```python
from build123d import *

# Parameters (mm, degrees)
ESQUISSE1_W             = 70
ESQUISSE1_H             = 30
BOSS_EXTRU_1_DEPTH      = 10
ESQUISSE2_R             = 0.8
ENL_V_MAT_EXTRU_1_DEPTH = 77.811457479
ESQUISSE3_R             = 1.025
ENL_V_MAT_EXTRU_2_DEPTH = 77.811457622
CONG_2_R                = 20


with BuildPart() as part:
    # Esquisse1 → Boss.-Extru.1 (new body)
    with BuildSketch(Plane.XY):
        with Locations((35, 15)):
            Rectangle(ESQUISSE1_W, ESQUISSE1_H)
    extrude(amount=BOSS_EXTRU_1_DEPTH)

    # Esquisse2 → Enlèv. mat.-Extru.1 (cut, through all)
    with BuildSketch(Plane.XY.offset(10)):
        with Locations((53.974554028, 20.976947928)):
            Circle(ESQUISSE2_R)
        with Locations((59.413465757, 18.443523524)):
            Circle(ESQUISSE2_R)
        with Locations((59.938911728, 12.466575596)):
            Circle(ESQUISSE2_R)
        with Locations((55.025445972, 9.023052072)):
            Circle(ESQUISSE2_R)
        with BuildLine():
            ThreePointArc((54.940833126, 19.980528702), (59.5, 15), (54.940833126, 10.019471298))
            add(Edge.make_bspline(
                [(48.86, 7.668533571), (51.540343022, 10.446024006), (54.940833126, 10.019471298)],
                knots=[0, 0, 0, 1, 1, 1], degree=2))
            ThreePointArc((48.86, 7.668533571), (28.5, 15), (48.86, 22.331466429))
            add(Edge.make_bspline(
                [(48.86, 22.331466429), (51.534478996, 19.459310032), (54.940833126, 19.980528702)],
                knots=[0, 0, 0, 1, 1, 1], degree=2))
        make_face()
    extrude(amount=-ENL_V_MAT_EXTRU_1_DEPTH, mode=Mode.SUBTRACT)

    # Esquisse3 → Enlèv. mat.-Extru.2 (cut, through all)
    with BuildSketch(Plane.XY.offset(10)):
        with Locations((5, 25)):
            Circle(ESQUISSE3_R)
        with Locations((65.771138483, 5)):
            Circle(ESQUISSE3_R)
        with Locations((65, 25)):
            Circle(ESQUISSE3_R)
    extrude(amount=-ENL_V_MAT_EXTRU_2_DEPTH, mode=Mode.SUBTRACT)

    # Congé2
    cong_2_edges = [part.edges().sort_by_distance(p)[0] for p in [
        (0, 0, 5),
    ]]
    fillet(cong_2_edges, radius=CONG_2_R)


solid = part.part
```
Part model, mm, in its own coordinate system. A direction names the side the tool comes from. Round coordinates to 2 decimals unless told otherwise and drop trailing zeros. Write each loop counter-clockwise with the first axis right and the second up, starting at its lowest first coordinate (ties: lowest second). Pieces come first, ordered by that corner, then holes.
Item 1: Which spindle directions (+Z, -Z, +X, -X, +Y, -Y) get a long thin tool onto all of the face, cutting with end or side? Do faces 1 (the cylindrical face through (59.5, 15.1, 5.1)), 2 (the flat face through (45, 0, 5)). Say none if no direction does.
Results:
face 1: +Z, -Z
face 2: +Z, -Z, +X, -X, -Y
Item 2: Cut at D-D, the plane y = 15. Give the cut face in (x, z), plus the area to 3 significant figures.
Results:
outline: (0.64, 0) - (28.5, 0) - (28.5, 10) - (0.64, 10) - close; (59.5, 0) - (70, 0) - (70, 10) - (59.5, 10) - close
area: 384 mm2
Item 3: Drop flat-ended pins along their axis: pin 1 Ø3 at (y, z) = (14, 6) entering from -X; pin 2 Ø1.3 at (x, y) = (55.03, 9.02) entering from -Z. Give the stop position or say it passes through.
Results:
pin 1: stops at x = 0.51
pin 2: passes through
Item 4: Probe L1, parallel to X at y = 21.5, z = 2.25; L2, parallel to X at y = 19.5, z = 9.25; L3, parallel to Y at x = 30, z = 8. List the from-to ranges inside material, lowest first.
Results:
L1: x = 0 to 30.51, 49.73 to 53.37, 54.58 to 70
L2: x = 0.01 to 29.42, 56.68 to 70
L3: y = 0 to 9.32, 20.68 to 30
Item 5: Cut at A-A, the plane x = 40. Give the cut face in (y, z).
Results:
outline: (0, 0) - (3.5, 0) - (3.5, 10) - (0, 10) - close; (26.5, 0) - (30, 0) - (30, 10) - (26.5, 10) - close
Item 6: Cut at C-C, the plane y = 25. Give the cut face in (x, z) (3 decimals), plus the area to 3 significant figures.
Results:
outline: (0, 0) - (3.975, 0) - (3.975, 10) - (0, 10) - close; (6.025, 0) - (34.321, 0) - (34.321, 10) - (6.025, 10) - close; (45.679, 0) - (63.975, 0) - (63.975, 10) - (45.679, 10) - close; (66.025, 0) - (70, 0) - (70, 10) - (66.025, 10) - close
area: 545 mm2
Item 7: Cut at B-B, the plane y = 5. Give the cut face in (x, z).
Results:
outline: (6.77, 0) - (34.32, 0) - (34.32, 10) - (6.77, 10) - close; (45.68, 0) - (64.75, 0) - (64.75, 10) - (45.68, 10) - close; (66.8, 0) - (70, 0) - (70, 10) - (66.8, 10) - close
Item 8: Two-plate mould, pull along X, no slides. Class faces 3 (the cylindrical face through (5.703, 6.014, 5.07)), 4 (the flat face through (27, 15, 0)), 5 (the cylindrical face through (60.68, 12.16, 5.07)): +X half, -X half, draft (parallel to the pull), parting line (faces both ways), or undercut.
Results:
face 3: -X half
face 4: draft
face 5: undercut
